from build123d import *

# Parameters (mm, degrees)
BOSS_EXTRUDE1_DEPTH     = 7.5
LPATTERN1_COUNT         = 8
LPATTERN1_PITCH         = 7
LPATTERN1_COL_COUNT     = 8
LPATTERN1_COL_PITCH     = 7
SHELL2_T                = -1
SKETCH3_W               = 0.5
SKETCH3_H               = 4.5
CUT_EXTRUDE2_DEPTH      = 15
CUT_EXTRUDE2_DEPTH_BACK = 8.5
SKETCH4_W               = 13
SKETCH4_H               = 2.5
BOSS_EXTRUDE2_DEPTH     = 1
SKETCH5_W               = 13
SKETCH5_H               = 2.5
BOSS_EXTRUDE3_DEPTH     = 1
SKETCH8_W               = 6
SKETCH8_H               = 15
BOSS_EXTRUDE5_DEPTH     = 2
LPATTERN2_COUNT         = 15
LPATTERN2_PITCH         = 7


with BuildPart() as part:
    # Sketch1 → Boss-Extrude1 (new body, symmetric)
    with BuildSketch(Plane.XY):
        Polygon((0, 0), (-3.5, 0), (-3.5, 4.5), (-3, 4.5), (-3, 22.5), (3, 22.5), (3, 4.5), (3.5, 4.5), (3.5, 0), align=None)
    boss_extrude1 = extrude(amount=BOSS_EXTRUDE1_DEPTH, both=True)

    # LPattern1: Boss-Extrude1 ×8
    with Locations(*[(i * LPATTERN1_PITCH, 0, 0) for i in range(1, LPATTERN1_COUNT)]):
        add(boss_extrude1)

    # LPattern1 col: Boss-Extrude1 ×8
    with Locations(*[(-i * LPATTERN1_COL_PITCH, 0, 0) for i in range(1, LPATTERN1_COL_COUNT)]):
        add(boss_extrude1)

    # Shell2
    shell2_openings = [part.faces().sort_by_distance(p)[0] for p in [
        (52.5, 2.25, 0),
        (-52.5, 2.25, 0),
    ]]
    offset(amount=SHELL2_T, openings=shell2_openings, kind=Kind.INTERSECTION)

    # Sketch3 → Cut-Extrude2 (cut, two sides)
    with BuildSketch(Plane.XY) as cut_extrude2_sk:
        with Locations((-52.25, 2.25)):
            Rectangle(SKETCH3_W, SKETCH3_H)
        with Locations((52.25, 2.25)):
            Rectangle(SKETCH3_W, SKETCH3_H)
    extrude(amount=CUT_EXTRUDE2_DEPTH, mode=Mode.SUBTRACT)
    extrude(cut_extrude2_sk.sketch, amount=-CUT_EXTRUDE2_DEPTH_BACK, mode=Mode.SUBTRACT)

    # Sketch4 → Boss-Extrude2 (add)
    with BuildSketch(Plane.ZY.offset(52)):
        with Locations((0, 2.25)):
            Rectangle(SKETCH4_W, SKETCH4_H)
    extrude(amount=-BOSS_EXTRUDE2_DEPTH)

    # Sketch5 → Boss-Extrude3 (add)
    with BuildSketch(Plane(origin=(52, 0, 0), x_dir=(0, 0, -1), z_dir=(1, 0, 0))):
        with Locations((0, 2.25)):
            Rectangle(SKETCH5_W, SKETCH5_H)
    extrude(amount=-BOSS_EXTRUDE3_DEPTH)

    # Sketch8 → Boss-Extrude5 (add)
    with BuildSketch(Plane(origin=(0, 22.5, 0), x_dir=(1, 0, 0), z_dir=(0, 1, 0))):
        with Locations((-49, 0)):
            Rectangle(SKETCH8_W, SKETCH8_H)
    boss_extrude5 = extrude(amount=BOSS_EXTRUDE5_DEPTH)

    # LPattern2: Boss-Extrude5 ×15
    with Locations(*[(i * LPATTERN2_PITCH, 0, 0) for i in range(1, LPATTERN2_COUNT)]):
        add(boss_extrude5)


solid = part.part
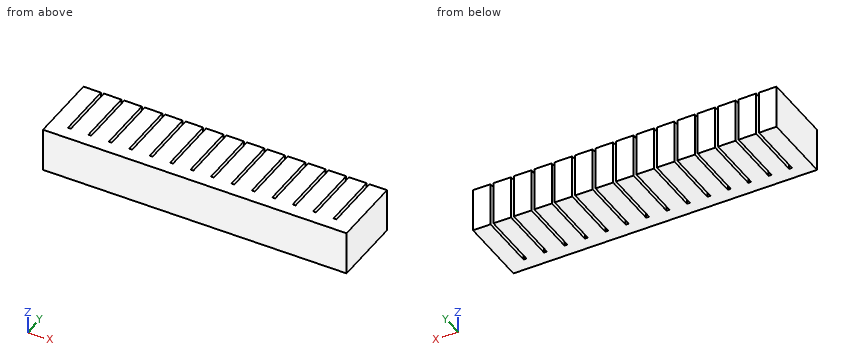
Design review of the part built by this model. Coordinates are the model's own, in mm. Coordinates: 2 decimals unless noted, no trailing zeros. Order: outer loops, then holes, each group sorted by start corner. A loop starts at its lowest first (then second) coordinate and runs counter-clockwise, first axis right, second up. Notation, with made-up numbers: M 68,37.25 L 125,37.25 A17 ccw 125,67.25 Z; hole C 28,-0.5 d5. An arc over 180 degrees is marked long. Use a Markdown table: item, result.
(1) Add section A-A (y = 2.5). Give the boundary of the cut face in (x, z).
Worked answers:
| item | result |
|---|---|
| outline | M -52,-7.5 L 52,-7.5 L 52,7.5 L -52,7.5 Z; hole M -51,-6.5 L 51,-6.5 L 51,6.5 L -51,6.5 Z |
(2) Add section B-B (x = -43). Give the boundary of the cut face in (y, z), then the cut area to 3 significant figures.
Worked answers:
| item | result |
|---|---|
| outline | M 0,-7.5 L 24.5,-7.5 L 24.5,7.5 L 0,7.5 Z; hole M 1,-6.5 L 21.5,-6.5 L 21.5,6.5 L 1,6.5 Z |
| area | 101 mm2 |
(3) Add section C-C (y = 19). Count the separate pieces of the cut face and the enclosed holes in it, then the cut area to 3 significant figures.
Worked answers:
| item | result |
|---|---|
| separate pieces | 15 |
| enclosed holes | 15 |
| area | 570 mm2 |
(4) Wall thickness on probe 1 along Y at (x, z) = (-25.5, 0.25); probe 2 along Z at (x, y) = (29, 19.5); probe 3 along X at (y, z) = (1.5, 1.25): over which ranges is each line inside the solid? List them lowest first.
Worked answers:
| item | result |
|---|---|
| probe 1 | y = 0 to 1, 3.5 to 24.5 |
| probe 2 | z = -7.5 to -6.5, 6.5 to 7.5 |
| probe 3 | x = -52 to -51, 51 to 52 |
(5) For P1, Ø0.8, axis at x = -10.5, z = -1, coming from the +Y side, flat-tipped, find the tip position at first contact; note if it passes through.
Worked answers:
| item | result |
|---|---|
| P1 | stops at y = 4.5 |
